```python
from build123d import *

# Parameters (mm, degrees)
BOSS_EXTRUDE1_DEPTH = 6.5


with BuildPart() as part:
    # Sketch1 → Boss-Extrude1 (new, symmetric)
    with BuildSketch(Plane(origin=(0, 0, 0), x_dir=(1, 0, 0), z_dir=(0, 1, 0))):
        with BuildLine():
            Line((0, 242), (0, -242))
            Line((0, -242), (-46, -242))
            Line((-46, -242), (-46, -232.5))
            Line((-46, -232.5), (-383.656025613, -232.5))
            ThreePointArc((-383.656025613, -232.5), (-417.305553076, -218.648136781), (-440.836676218, -190.891136639))
            ThreePointArc((-440.836676218, -190.891136639), (-485.999569897, -0.605349387), (-441.377653297, 189.808022923))
            ThreePointArc((-441.377653297, 189.808022923), (-412.985038869, 220.962652578), (-372.443194837, 232.5))
            Line((-372.443194837, 232.5), (-46, 232.5))
            Line((-46, 232.5), (-46, 242))
            Line((-46, 242), (0, 242))
        make_face()
    extrude(amount=BOSS_EXTRUDE1_DEPTH, both=True)


solid = part.part
```
Check sheet for the modelled part. Datum: model origin and axes. Units: mm. A direction names the side the tool comes from. Coordinates: 2 decimals unless noted, no trailing zeros. Loops run counter-clockwise (first coordinate to the right, second up) from the corner with the lowest first, then second, coordinate; pieces in that order, holes last. Notation, with made-up numbers: M -33.75,56.5 L 5.25,56.5 A18 ccw 5.25,91.5 Z; hole C -7,-28.5 d4. An arc over 180 degrees is marked long. Answer as a JSON object with one key per item and string values.
1. Sectioned sample at B-B on x = -129. Record the cut outline in (y, z).
Outcome:
{"outline": "M -6.5,-232.5 L 6.5,-232.5 L 6.5,232.5 L -6.5,232.5 Z"}
2. Sectioned sample at C-C on z = 83. Record the cut outline in (x, y).
Outcome:
{"outline": "M -477.84,-6.5 L 0,-6.5 L 0,6.5 L -477.84,6.5 Z"}
3. Depth check by flat-ended pin: P1, Ø6.5, axis at x = -255, y = 2, coming from the -Z side; P2, Ø3, axis at y = 1, z = -103, coming from the -X side; P3, Ø6.5, axis at x = -265.5, y = 0, coming from the +Z side. Enter the tip coordinate at first touch or a pass-through.
Outcome:
{"P1": "z = -232.5", "P2": "x = -473.73", "P3": "z = 232.5"}
4. Sectioned sample at A-A on y = 3.5. Record the cut outline in (x, z).
Outcome:
{"outline": "M -441.38,-189.81 A77 ccw -372.44,-232.5 L -46,-232.5 L -46,-242 L 0,-242 L 0,242 L -46,242 L -46,232.5 L -383.66,232.5 A77 ccw -440.84,190.89 A426 ccw Z"}
5. Access from +Z, -Z, +X, -X, +Y, -Y to the whole of each face (thin tool, end or side, straight path). Record for faces 1 (the flat face through (-212, 0, 232.5)), 2 (the flat face through (-212, 0, -232.5)), 3 (the flat face through (-240, 6.5, -3)).
Outcome:
{"face 1": "+Z, -X, +Y, -Y", "face 2": "-Z, -X, +Y, -Y", "face 3": "+Z, -Z, +X, -X, +Y"}
6. Scan lines: L1, parallel to Z at x = -237, y = -1; L2, parallel to X at y = 2.75, z = 3; L3, parallel to X at y = -5, z = -142.5. Record each from-to range of solid material in increasing order. Write a range as from..to.
Outcome:
{"L1": "-232.5..232.5", "L2": "-485.99..0", "L3": "-461.46..0"}
